The model under review builds one solid part; all positions refer to its coordinate system, in mm. Face numbers are marked on the shaded views. Round coordinates to 2 decimals unless told otherwise and drop trailing zeros. Order: outer loops, then holes, each group sorted by start corner. A loop starts at its lowest first (then second) coordinate and runs counter-clockwise, first axis right, second up.
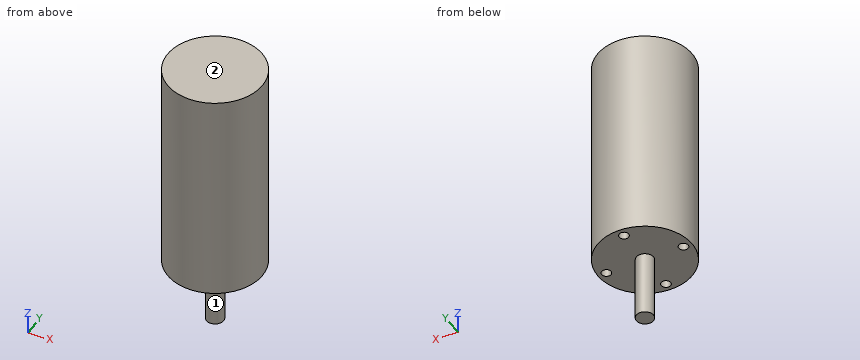
```python
from build123d import *

# Parameters (mm, degrees)
SKETCH1_R               = 10.999999971
SKETCH1_R_2             = 2
BOSS_EXTRUDE4_DEPTH     = 50.1
SKETCH1_6_R             = 2
BOSS_EXTRUDE5_DEPTH     = 15.3
ADVANCEDHOLE1_OUTLINE_R = 1.1
ADVANCEDHOLE1_DEPTH     = 2


# Read off the part's stored shape, not the designer's step: AdvancedHole1
with BuildPart() as part:
    # Sketch1 → Boss-Extrude4 (new body)
    # profile 1 of 2: a face of its own
    with BuildSketch(Plane.XY):
        Circle(SKETCH1_R)
        Circle(SKETCH1_R_2, mode=Mode.SUBTRACT)
    # profile 2 of 2: a face of its own
    with BuildSketch(Plane.XY):
        Circle(SKETCH1_R_2)
    extrude(amount=BOSS_EXTRUDE4_DEPTH)

    # Sketch1<6> → Boss-Extrude5 (add)
    with BuildSketch(Plane.XY):
        Circle(SKETCH1_6_R)
    extrude(amount=-BOSS_EXTRUDE5_DEPTH)

    # AdvancedHole1 outline → AdvancedHole1 (cut)
    with BuildSketch(Plane.XY):
        with Locations((0, -9)):
            Circle(ADVANCEDHOLE1_OUTLINE_R)
        with Locations((-9, 0)):
            Circle(ADVANCEDHOLE1_OUTLINE_R)
        with Locations((0, 9)):
            Circle(ADVANCEDHOLE1_OUTLINE_R)
        with Locations((9, 0)):
            Circle(ADVANCEDHOLE1_OUTLINE_R)
    extrude(amount=ADVANCEDHOLE1_DEPTH, mode=Mode.SUBTRACT)


solid = part.part
```
(1) Consider section D-D (y = -9). Write out the cut boundary in (x, z).
Data:
outline: (-6.32, 0) - (-1.1, 0) - (-1.1, 2) - (1.1, 2) - (1.1, 0) - (6.32, 0) - (6.32, 50.1) - (-6.32, 50.1) - close
(2) To check wall thickness, follow probe 1 along Y at (x, z) = (0, 0.55); probe 2 along Z at (x, y) = (-2.75, 4.25); probe 3 along Y at (x, z) = (-9.25, 1). State the ranges of each line that lie inside material, in increasing order.
Data:
probe 1: y = -11 to -10.1, -7.9 to 7.9, 10.1 to 11
probe 2: z = 0 to 50.1
probe 3: y = -5.95 to -1.07, 1.07 to 5.95
(3) Consider section C-C (z = 26). Write out the cut boundary in (x, y).
Data:
outline: circle Ø22 at (0, 0)
(4) Insertion check: pin 1 (1.8 mm diameter, centred on x = 0, y = 8.5, fed in from -Z); pin 2 (10 mm diameter, centred on y = -5.5, z = 14, fed in from +X); pin 3 (5 mm diameter, centred on y = -8, z = 39.5, fed in from +X). Each pin has a flat end and moves straight along its axis. Give the tip position at first contact, or say it passes through.
Data:
pin 1: stops at z = 0
pin 2: stops at x = 10.99
pin 3: stops at x = 9.53
(5) Draft analysis for pull direction X (two halves, no side actions). For the marked faces 1 and 2, state which applies: pulls with the +X half, pulls with the -X half, needs draft (parallel to the pull), parting line crosses it, or undercut.
Data:
face 1: parting line crosses it
face 2: needs draft
(6) Consider section A-A (x = 0). Write out the cut boundary in (y, z), and give its area (3 significant figures).
Data:
outline: (-11, 0) - (-10.1, 0) - (-10.1, 2) - (-7.9, 2) - (-7.9, 0) - (-2, 0) - (-2, -15.3) - (2, -15.3) - (2, 0) - (7.9, 0) - (7.9, 2) - (10.1, 2) - (10.1, 0) - (11, 0) - (11, 50.1) - (-11, 50.1) - close
area: 1,150 mm2
